```python
from build123d import *

# Parameters (mm, degrees)
SKETCH1_W           = 20
SKETCH1_H           = 80
BOSS_EXTRUDE1_DEPTH = 10
SKETCH3_W           = 50
SKETCH3_H           = 20
BOSS_EXTRUDE2_DEPTH = 10


with BuildPart() as part:
    # Sketch1 → Boss-Extrude1 (new body)
    with BuildSketch(Plane(origin=(0, 0, 0), x_dir=(1, 0, 0), z_dir=(0, 1, 0))):
        Rectangle(SKETCH1_W, SKETCH1_H)
    extrude(amount=BOSS_EXTRUDE1_DEPTH)

    # Sketch3 → Boss-Extrude2 (add)
    with BuildSketch(Plane(origin=(0, 10, 0), x_dir=(1, 0, 0), z_dir=(0, 1, 0))):
        with Locations((15, -50)):
            Rectangle(SKETCH3_W, SKETCH3_H)
    extrude(amount=-BOSS_EXTRUDE2_DEPTH)


solid = part.part
```
CAD build for the part. Positions are in the model's coordinates, mm. A direction names the side the tool comes from. Round coordinates to 2 decimals unless told otherwise and drop trailing zeros. Loops run counter-clockwise (first coordinate to the right, second up) from the corner with the lowest first, then second, coordinate; pieces in that order, holes last. Notation, with made-up numbers: M -16,-25.75 L 31,-25.75 A22 cw 31,4.25 Z; hole C 88.5,51 d4. An arc over 180 degrees is marked long. Use a Markdown table: item, result. Add a question column.
(1) Drill centre lines: line 1 (X direction, y = 1, z = 6.5); line 2 (Z direction, x = 31.5, y = 3.75). Where is each one in solid material? Low to high.
(2) Flat gauge pin, fed straight in: pin 1 (1 mm diameter, centred on y = 1.5, z = 3, fed in from +X). Where does the tip first touch, or does it go through?
(3) Cut at B-B (x = 21). Give the cut face in (y, z).
(4) Cut at C-C (z = -3.5). Give the cut face in (x, y).
(5) Which spindle directions (+Z, -Z, +X, -X, +Y, -Y) get a long thin tool onto all of the face, cutting with end or side? Do faces 1 (the face through (4, 10, 20)), 2 (the face through (25, 5, 40)). Say none if no direction does.
(6) Cut at A-A (y = 6.5). Give the cut face in (x, z), and give its area (3 significant figures).
Geometry says:
| question | item | result |
|---|---|---|
| 1 | line 1 | x = -10 to 10 |
| 1 | line 2 | z = 40 to 60 |
| 2 | pin 1 | stops at x = 10 |
| 3 | outline | M 0,40 L 10,40 L 10,60 L 0,60 Z |
| 4 | outline | M -10,0 L 10,0 L 10,10 L -10,10 Z |
| 5 | face 1 | +Z, -Z, +X, -X, +Y |
| 5 | face 2 | -Z, +X, +Y, -Y |
| 6 | outline | M -10,-40 L 10,-40 L 10,40 L 40,40 L 40,60 L -10,60 Z |
| 6 | area | 2,600 mm² |
